Could you check a few things on this model? Use its own coordinates, in mm. A direction names the side the tool comes from. Coordinates: 2 decimals unless noted, no trailing zeros. Order: outer loops, then holes, each group sorted by start corner. A loop starts at its lowest first (then second) coordinate and runs counter-clockwise, first axis right, second up.
Autodesk Inventor part; units mm, degrees
ref_plane "YZ Plane" through (0, 0, 0) normal (1, 0, 0) x (0, 1, 0)
ref_plane "XZ Plane" through (0, 0, 0) normal (0, 1, 0) x (-1, 0, 0)
ref_plane "XY Plane" through (0, 0, 0) normal (0, 0, 1) x (1, 0, 0)
sketch "Náčrt1" plane through (0, 0, 0) normal (0, 1, 0) x (-1, 0, 0)
  line L0 (-2.8868, 0) -> (-1.4434, 2.5)
  line L1 (-1.4434, 2.5) -> (1.4434, 2.5)
  line L2 (1.4434, 2.5) -> (2.8868, 0)
  line L3 (2.8868, 0) -> (1.4434, -2.5)
  line L4 (1.4434, -2.5) -> (-1.4434, -2.5)
  line L5 (-1.4434, -2.5) -> (-2.8868, 0)
  point P0 (0, 0)
  point P1 (0, 0)
  dimension "d0" = 5
extrude "Vysunutí1" add sketch "Náčrt1" along normal blind 20
sketch "Náčrt2" plane through (0, 20, 0) normal (0, 1, 0) x (1, 0, 0)
  circle A0 centre (0, 0) radius 1.5
  dimension "d3" = 3
extrude "Vysunutí2" cut sketch "Náčrt2" against normal blind 8
thread "Závit1"
sketch "Náčrt3" plane through (0, 0, 0) normal (0, -1, 0) x (1, 0, 0)
  circle A0 centre (0, 0) radius 1.5
extrude "Vysunutí3" add sketch "Náčrt3" along normal blind 8
thread "Závit2"
properties part number "m3x20mm distanční sloupek"
Item 1: Suppose I cut it at A-A (z = -0.4). List the corners of the cut face in (x, y) for me, and give its area (3 significant figures).
Item 2: Suppose I cut it at B-B (x = 1). List the corners of the cut face in (y, z) for me, and give its area (3 significant figures).
Item 3: Which directions (+Z, -Z, +X, -X, +Y, -Y) give clear straight access to the entire face, cutting with the end or side of a thin tool? Please do faces 1 (the face through (-1.5, -3.94, -0.07)), 2 (the face through (0, -8, 0)).
Item 4: Thinking about a two-plate mould opening in Z: for faces 3 (the face through (-1.24, 20, 1.15)), 4 (the face through (2.155, 9.86, -1.267)), 5 (the face through (-1.5, 16.06, -0.07)), 6 (the face through (0, 12, 0)), which applies, +Z half, -Z half, draft (parallel to the pull), parting line (faces both ways), or undercut?
Item 5: I need wall thicknesses on line 1 (Z direction, x = 0, y = 17.5); line 2 (Y direction, x = 1.3, z = -1.25); line 3 (Y direction, x = -1.4, z = 0). Which ranges of each line are inside material? Lowest first, please.
Item 6: For pin 1 Ø0.9 at (x, z) = (0, 0.5) entering from +Y; pin 2 Ø1.5 at (y, z) = (-4, 1.5) entering from +X, each with a flat end and sliding along its axis, tell me the tip position at first contact or that it passes through.
Geometry results:
1. outline: (-2.66, 0) - (-1.45, 0) - (-1.45, -8) - (1.45, -8) - (1.45, 0) - (2.66, 0) - (2.66, 20) - (1.45, 20) - (1.45, 12) - (-1.45, 12) - (-1.45, 20) - (-2.66, 20) - close
1. area: 106 mm2
2. outline: (-8, -1.12) - (0, -1.12) - (0, -2.5) - (20, -2.5) - (20, -1.12) - (12, -1.12) - (12, 1.12) - (20, 1.12) - (20, 2.5) - (0, 2.5) - (0, 1.12) - (-8, 1.12) - close
2. area: 100 mm2
3. face 1: -Y
3. face 2: +Z, -Z, +X, -X, -Y
4. face 3: draft
4. face 4: -Z half
4. face 5: undercut
4. face 6: undercut
5. line 1: z = -2.5 to -1.5, 1.5 to 2.5
5. line 2: y = 0 to 20
5. line 3: y = -8 to 12
6. pin 1: stops at y = 12
6. pin 2: stops at x = 1.3
